Part model, mm, in its own coordinate system. A direction names the side the tool comes from. Coordinates: 2 decimals unless noted, no trailing zeros. Order: outer loops, then holes, each group sorted by start corner. A loop starts at its lowest first (then second) coordinate and runs counter-clockwise, first axis right, second up. Notation, with made-up numbers: (-19.5, 16.5) - (31.5, 16.5) arc R30 cw to (31.5, 38.5) - close; hole circle Ø8 at (9.25, 15). An arc over 180 degrees is marked (long way). Use a Markdown table: item, result. Add a question column.
1) Drop flat-ended pins along their axis: P1, Ø1.1, axis at x = -1.5, y = 1, coming from the -Z side; P2, Ø1.2, axis at x = 0, z = 0, coming from the -Y side; P3, Ø0.8, axis at y = 1, z = -1.5, coming from the +X side. Give the stop position or say it passes through.
2) Two-plate mould, pull along X, no slides. Class faces 1 (the face through (-0.5, 0.7, -1.5)), 2 (the face through (0, 7, 2)), 3 (the face through (2, 2.15, 1)): +X half, -X half, draft (parallel to the pull), parting line (faces both ways), or undercut.
3) Wall check: L1, parallel to Y at x = -0.5, z = -2.25; L2, parallel to Y at x = -0.5, z = 0.25; L3, parallel to Z at x = 1.25, y = 11.75. Give the ranges that are in metal, low to high. Write a range as [from, to].
4) Saw through at A-A on z = 0. List the corners of the cut face in (x, y).
5) Saw through at D-D on x = -3. List the corners of the cut face in (y, z).
6) Saw through at B-B on x = 0. List the corners of the cut face in (y, z), then the cut area to 3 significant figures.
7) Tool access for faces 4 (the face through (-2, 1, 0)), 5 (the face through (0, 12.15, 0)): list every direction of +Z, -Z, +X, -X, +Y, -Y with a clear straight run to the whole face (end or side of a thin tool).
8) Saw through at C-C on y = 3. List the corners of the cut face in (x, z).
```python
from build123d import *

# Parameters (mm, degrees)
SKETCH_1_R          = 3.15
EXTRUDE_1_DEPTH     = 2.15
SKETCH_2_R          = 2
EXTRUDE_2_DEPTH     = 10
CUT_EXTRUDE_1_DEPTH = 1.5


with BuildPart() as part:
    # 草图1 → 凸台-拉伸1 (new body)
    with BuildSketch(Plane(origin=(0, 0, 0), x_dir=(1, 0, 0), z_dir=(0, 1, 0))):
        Circle(SKETCH_1_R)
    extrude(amount=EXTRUDE_1_DEPTH)

    # 草图2 → 凸台-拉伸2 (add)
    with BuildSketch(Plane(origin=(0, 2.15, 0), x_dir=(1, 0, 0), z_dir=(0, 1, 0))):
        Circle(SKETCH_2_R)
    extrude(amount=EXTRUDE_2_DEPTH)

    # 草图3 → 切除-拉伸1 (cut)
    with BuildSketch(Plane.XZ):
        with BuildLine():
            Line((-0.5, 1), (-0.5, 2))
            Line((-0.5, 2), (0.5, 2))
            Line((0.5, 2), (0.5, 1))
            ThreePointArc((0.5, 1), (0.646446609, 0.646446609), (1, 0.5))
            Line((1, 0.5), (2, 0.5))
            Line((2, 0.5), (2, -0.5))
            Line((2, -0.5), (1, -0.5))
            ThreePointArc((1, -0.5), (0.646446609, -0.646446609), (0.5, -1))
            Line((0.5, -1), (0.5, -2))
            Line((0.5, -2), (-0.5, -2))
            Line((-0.5, -2), (-0.5, -1))
            ThreePointArc((-0.5, -1), (-0.646446609, -0.646446609), (-1, -0.5))
            Line((-1, -0.5), (-2, -0.5))
            Line((-2, -0.5), (-2, 0.5))
            Line((-2, 0.5), (-1, 0.5))
            ThreePointArc((-1, 0.5), (-0.646446609, 0.646446609), (-0.5, 1))
        make_face()
    extrude(amount=-CUT_EXTRUDE_1_DEPTH, mode=Mode.SUBTRACT)


solid = part.part
```
Results are:
| question | item | result |
|---|---|---|
| 1 | P1 | z = -3 |
| 1 | P2 | y = 1.5 |
| 1 | P3 | x = 2.95 |
| 2 | face 1 | undercut |
| 2 | face 2 | parting line |
| 2 | face 3 | draft |
| 3 | L1 | [0, 2.15] |
| 3 | L2 | [1.5, 12.15] |
| 3 | L3 | [-1.56, 1.56] |
| 4 | outline | (-3.15, 0) - (-2, 0) - (-2, 1.5) - (2, 1.5) - (2, 0) - (3.15, 0) - (3.15, 2.15) - (2, 2.15) - (2, 12.15) - (-2, 12.15) - (-2, 2.15) - (-3.15, 2.15) - close |
| 5 | outline | (0, -0.96) - (2.15, -0.96) - (2.15, 0.96) - (0, 0.96) - close |
| 6 | outline | (0, -3.15) - (2.15, -3.15) - (2.15, -2) - (12.15, -2) - (12.15, 2) - (2.15, 2) - (2.15, 3.15) - (0, 3.15) - (0, 2) - (1.5, 2) - (1.5, -2) - (0, -2) - close |
| 6 | area | 47.5 mm2 |
| 7 | face 4 | -Y |
| 7 | face 5 | +Z, -Z, +X, -X, +Y |
| 8 | outline | circle Ø4 at (0, 0) |
